Verification items for the finished model (mm, model axes). A direction names the side the tool comes from. Coordinates: 2 decimals unless noted, no trailing zeros. Loops run counter-clockwise (first coordinate to the right, second up) from the corner with the lowest first, then second, coordinate; pieces in that order, holes last. Notation, with made-up numbers: (73, -16.5) -> (78, -16.5) arc R20 cw to (78, 6.5) -> close; hole circle Ø1 at (-15, 38.5). An arc over 180 degrees is marked (long way). Answer as a JSON object with one key per item and string values. Group by question number.
Q1. Gauge pin test, flat ends, axial feed: pin 1 Ø1 at (y, z) = (3, -6.5) entering from +X; pin 2 Ø3 at (x, y) = (-6.5, 5.5) entering from +Z; pin 3 Ø7 at (x, z) = (0, 0) entering from -Y. Record the tip position at first contact, or that the pin passes through.
Q2. Scan lines: L1, parallel to Z at x = 0, y = 2.4; L2, parallel to Z at x = 0, y = 1.25; L3, parallel to X at y = 4.25, z = 0.75. Record each from-to range of solid material in increasing order.
Q3. Cross-section at B-B on y = 0.75. Record the boundary of the cut face in (x, z).
Q4. Cross-section at A-A on y = 2.5. Record the boundary of the cut face in (x, z).
Q5. Set-up check for faces 1 (the flat face through (-2, 3, -7.4)), 2 (the cylindrical face through (5.723, 1.606, -1.802)), 3 (the cylindrical face through (8.584, 5.226, -2.703)): record each of +Z, -Z, +X, -X, +Y, -Y from which the full face is reachable in a straight line by a thin tool's end or side.
Q6. Release check for a two-part mould opening along Y. For faces 4 (the cylindrical face through (-6.633, 2.26, -6.083)), 5 (the cylindrical face through (4.032, 4.014, -6.324)), 6 (the flat face through (3, 0, -6)), 7 (the flat face through (2, 5, -7.4)) record: released by +Y, released by -Y, zero draft, split by the parting line, or undercut.
```python
from build123d import *
from OCP.BRepFilletAPI import BRepFilletAPI_MakeChamfer

# Parameters (mm, degrees)
CHAMFER1_SIZE  = 0.25
CHAMFER1_SIZE2 = 0.304621849


with BuildPart() as part:
    # Sketch1 → Revolve1 (revolve)
    with BuildSketch(Plane.XY, mode=Mode.PRIVATE) as revolve1_sk:
        with BuildLine():
            Line((-6, 0), (-7.5, 0))
            Line((-7.5, 0), (-9, 1.5))
            Line((-9, 1.5), (-9, 3))
            Line((-9, 3), (-7.5, 3))
            Line((-7.5, 3), (-7.5, 5))
            Line((-7.5, 5), (-9, 5))
            Line((-9, 5), (-9, 5.75))
            ThreePointArc((-9, 5.75), (-4.515597967, 6.312175605), (0, 6.5))
            Line((0, 6.5), (0, 5))
            add(Edge.make_bspline(
                [(0, 5), (-6, 5), (-6, 3)],
                knots=[1.570796327, 1.570796327, 1.570796327, 3.141592654, 3.141592654, 3.141592654], degree=2, weights=[1, 0.707106781, 1]))
            Line((-6, 3), (-6, 0))
        make_face()
    revolve(revolve1_sk.sketch.rotate(Axis((0, -1000, 0), (0, 1, 0)), 180), axis=Axis((0, -1000, 0), (0, 1, 0)))

    # Chamfer1: one chamfer whose edges measure the first distance from different faces: ONE call of the kernel's chamfer builder (chamfer() names one face for all edges)
    chamfer1_edges_1 = [part.edges().sort_by_distance(p)[0] for p in [
        (-9, 5.75, 0),
    ]]
    chamfer1_side_1 = [part.faces().sort_by_distance(p)[0] for p in [
        (-4.515597967, 6.312175605, 0),
    ]]
    chamfer1_edges_2 = [part.edges().sort_by_distance(p)[0] for p in [
        (-6, 0, 0),
    ]]
    chamfer1 = BRepFilletAPI_MakeChamfer(part.part.solid().wrapped)
    for e in chamfer1_edges_1:
        chamfer1.Add(CHAMFER1_SIZE, CHAMFER1_SIZE2, e.wrapped, chamfer1_side_1[0].wrapped)  # the first distance lies on this face
    for e in chamfer1_edges_2:
        chamfer1.Add(CHAMFER1_SIZE, e.wrapped)
    add(Compound.cast(chamfer1.Shape()), mode=Mode.REPLACE)


solid = part.part
```
Computed values:
{
 "1": {"pin 1": "stops at x = 6.71", "pin 2": "stops at z = 7.48", "pin 3": "stops at y = 4.62"},
 "2": {"L1": "z = -9 to -6, 6 to 9", "L2": "z = -8.75 to -6, 6 to 8.75", "L3": "x = -7.46 to -4.62, 4.62 to 7.46"},
 "3": {"outline": "circle Ø16.5 at (0, 0); hole circle Ø12 at (0, 0)"},
 "4": {"outline": "circle Ø18 at (0, 0); hole circle Ø12 at (0, 0)"},
 "5": {"face 1": "none", "face 2": "-Y", "face 3": "+Y, -Y"},
 "6": {"face 4": "zero draft", "face 5": "undercut", "face 6": "released by -Y", "face 7": "undercut"}
}
